Geometry check sheet. Reference: drawing and pictorial views, mm from the part's lowest x, y, z. Give positions to 0.01 mm unless a question says otherwise; leave off trailing zeros. Write each loop counter-clockwise with the first axis right and the second up, starting at its lowest first coordinate (ties: lowest second). Pieces come first, ordered by that corner, then holes. Notation, with made-up numbers: (74.25, 18.5) -> (105.25, 18.5) arc R11 ccw to (105.25, 36.5) -> close; hole circle Ø5 at (5, -20). An arc over 180 degrees is marked (long way). Return JSON: item names as keys, results as strings.
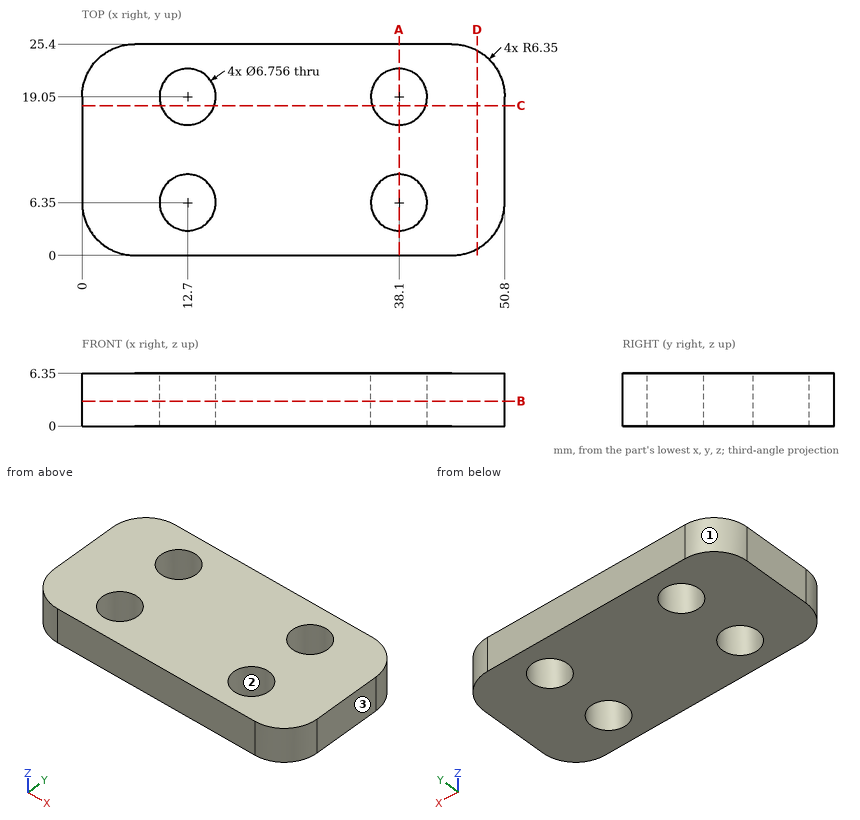
(1) Thickness scan on L1, parallel to Y at x = 12.7, z = 1.75; L2, parallel to X at y = 19.05, z = 4.75; L3, parallel to X at y = 21.25, z = 2.5 (1 decimal). Record the ranges inside material, lowest first.
Reply:
{"L1": "0 to 2.97, 9.73 to 15.67, 22.43 to 25.4", "L2": "0 to 9.32, 16.08 to 34.72, 41.48 to 50.8", "L3": "0.4 to 10.1, 15.3 to 35.5, 40.7 to 50.4"}
(2) Cross-section at A-A on x = 38.1. Enter the section's corners in (y, z).
Reply:
{"outline": "(0, 0) -> (2.97, 0) -> (2.97, 6.35) -> (0, 6.35) -> close; (9.73, 0) -> (15.67, 0) -> (15.67, 6.35) -> (9.73, 6.35) -> close; (22.43, 0) -> (25.4, 0) -> (25.4, 6.35) -> (22.43, 6.35) -> close"}
(3) Release check for a two-part mould opening along X. For the marked faces 1, 2 and 3 record: pulls with the +X half, pulls with the -X half, needs draft (parallel to the pull), parting line crosses it, or undercut.
Reply:
{"face 1": "pulls with the -X half", "face 2": "undercut", "face 3": "pulls with the +X half"}
(4) Cross-section at B-B on z = 3. Enter the section's corners in (x, y).
Reply:
{"outline": "(0, 6.35) arc R6.35 ccw to (6.35, 0) -> (44.45, 0) arc R6.35 ccw to (50.8, 6.35) -> (50.8, 19.05) arc R6.35 ccw to (44.45, 25.4) -> (6.35, 25.4) arc R6.35 ccw to (0, 19.05) -> close; hole circle Ø6.76 at (12.7, 6.35); hole circle Ø6.76 at (12.7, 19.05); hole circle Ø6.76 at (38.1, 6.35); hole circle Ø6.76 at (38.1, 19.05)"}
(5) Depth check by flat-ended pin: pin 1 Ø6 at (x, y) = (38.1, 6.35) entering from +Z; pin 2 Ø1.5 at (y, z) = (21.5, 2.5) entering from -X. Enter the tip coordinate at first touch or a pass-through.
Reply:
{"pin 1": "through", "pin 2": "x = 0.23"}
(6) Cross-section at C-C on y = 18. Enter the section's corners in (x, z).
Reply:
{"outline": "(0, 0) -> (9.49, 0) -> (9.49, 6.35) -> (0, 6.35) -> close; (15.91, 0) -> (34.89, 0) -> (34.89, 6.35) -> (15.91, 6.35) -> close; (41.31, 0) -> (50.8, 0) -> (50.8, 6.35) -> (41.31, 6.35) -> close"}
(7) Cross-section at D-D on x = 47.5. Enter the section's corners in (y, z).
Reply:
{"outline": "(0.78, 0) -> (24.62, 0) -> (24.62, 6.35) -> (0.78, 6.35) -> close"}
